```python
from build123d import *

# Parameters (mm, degrees)
EXTRUDE_1_DEPTH          = 5
EXTRUDE_2_DEPTH          = 15
EXTRUDE_2_DEPTH_BACK     = 5
SKETCH_3_R               = 3
CUT_EXTRUDE_1_DEPTH      = 3
SKETCH_4_R               = 2.1
CUT_EXTRUDE_2_DEPTH      = 10
CUT_EXTRUDE_3_DEPTH      = 86.718512573
CUT_EXTRUDE_3_DEPTH_BACK = 86.718512573
SKETCH_5_W               = 30
SKETCH_5_H               = 10
SKETCH_5_W_2             = 27.91179781
FILLET_1_R               = 3
CUT_EXTRUDE_4_DEPTH      = 88.407093534
CUT_EXTRUDE_4_DEPTH_BACK = 88.407093534
FILLET_2_R               = 3


with BuildPart() as part:
    # 草图1 → 凸台-拉伸1 (new body)
    with BuildSketch(Plane(origin=(0, 0, 0), x_dir=(1, 0, 0), z_dir=(0, 1, 0))):
        Polygon((0, 44.204391892), (-30, 44.204391892), (-30, -33.795608108), (0, -33.795608108), (30, -33.795608108), (30, 44.204391892), align=None)
    extrude(amount=EXTRUDE_1_DEPTH)

    # 草图2 → 凸台-拉伸2 (add, two sides: drawn at the far end of the back side and taken through both)
    with BuildSketch(Plane(origin=(0, 5, 0), x_dir=(1, 0, 0), z_dir=(0, 1, 0)).offset(-EXTRUDE_2_DEPTH_BACK)):
        Polygon((-30, -33.795608108), (-34, -33.795608108), (-34, 48.204391892), (34, 48.204391892), (34, -33.795608108), (30, -33.795608108), (30, 44.204391892), (-30, 44.204391892), align=None)
    extrude(amount=EXTRUDE_2_DEPTH + EXTRUDE_2_DEPTH_BACK)

    # 草图3 → 切除-拉伸1 (cut)
    with BuildSketch(Plane(origin=(0, 5, 0), x_dir=(1, 0, 0), z_dir=(0, 1, 0))):
        with Locations(Location((-20, 31.204391892, 0), (0, 0, 270))):
            Circle(SKETCH_3_R)
        with Locations(Location((20, 31.204391892, 0), (0, 0, 270))):
            Circle(SKETCH_3_R)
        with Locations(Location((-20, -18.795608108, 0), (0, 0, 270))):
            Circle(SKETCH_3_R)
        with Locations(Location((20, -18.795608108, 0), (0, 0, 270))):
            Circle(SKETCH_3_R)
    extrude(amount=-CUT_EXTRUDE_1_DEPTH, mode=Mode.SUBTRACT)

    # 草图4 → 切除-拉伸2 (cut)
    with BuildSketch(Plane(origin=(0, 2, 0), x_dir=(1, 0, 0), z_dir=(0, 1, 0))):
        with Locations(Location((-20, 31.204391892, 0), (0, 0, 270))):
            Circle(SKETCH_4_R)
        with Locations(Location((20, 31.204391892, 0), (0, 0, 270))):
            Circle(SKETCH_4_R)
        with Locations(Location((20, -18.795608108, 0), (0, 0, 270))):
            Circle(SKETCH_4_R)
        with Locations(Location((-20, -18.795608108, 0), (0, 0, 270))):
            Circle(SKETCH_4_R)
    extrude(amount=-CUT_EXTRUDE_2_DEPTH, mode=Mode.SUBTRACT)

    # 草图5 → 切除-拉伸3 (cut, two sides: drawn at the far end of the back side and taken through both)
    with BuildSketch(Plane.ZY.offset(34).offset(-CUT_EXTRUDE_3_DEPTH_BACK)):
        with Locations((-26.680193, 12)):
            Rectangle(SKETCH_5_W, SKETCH_5_H)
        with Locations((15.275705905, 12)):
            Rectangle(SKETCH_5_W_2, SKETCH_5_H)
    extrude(amount=CUT_EXTRUDE_3_DEPTH + CUT_EXTRUDE_3_DEPTH_BACK, mode=Mode.SUBTRACT)

    # 圆角1
    fillet_1_edges = [part.edges().sort_by_distance(p)[0] for p in [
        (-32, 17, -41.680193),
        (32, 17, -41.680193),
        (-32, 17, -11.680193),
        (32, 17, -11.680193),
        (-32, 7, -11.680193),
        (32, 7, -11.680193),
        (-32, 7, -41.680193),
        (32, 7, -41.680193),
        (-32, 17, 1.319807),
        (32, 17, 1.319807),
        (-32, 17, 29.23160481),
        (32, 17, 29.23160481),
        (-32, 7, 29.23160481),
        (32, 7, 29.23160481),
        (-32, 7, 1.319807),
        (32, 7, 1.319807),
    ]]
    fillet(fillet_1_edges, radius=FILLET_1_R)

    # 草图6 → 切除-拉伸4 (cut, two sides: drawn at the far end of the back side and taken through both)
    with BuildSketch(Plane.XY.offset(-44.204391892).offset(-CUT_EXTRUDE_4_DEPTH_BACK)):
        Polygon((0, 18), (-26, 18), (-26, 8), (26, 8), (26, 18), align=None)
    extrude(amount=CUT_EXTRUDE_4_DEPTH + CUT_EXTRUDE_4_DEPTH_BACK, mode=Mode.SUBTRACT)

    # 圆角2
    fillet_2_edges = [part.edges().sort_by_distance(p)[0] for p in [
        (26, 18, -46.204391892),
        (26, 8, -46.204391892),
        (-26, 8, -46.204391892),
        (-26, 18, -46.204391892),
    ]]
    fillet(fillet_2_edges, radius=FILLET_2_R)


solid = part.part
```
Design review of the part built by this model. Coordinates are the model's own, in mm. A direction names the side the tool comes from. Round coordinates to 2 decimals unless told otherwise and drop trailing zeros. Order: outer loops, then holes, each group sorted by start corner. A loop starts at its lowest first (then second) coordinate and runs counter-clockwise, first axis right, second up. Notation, with made-up numbers: (37.25, 59.25) - (59.25, 59.25) arc R11 cw to (59.25, 69.25) - close; hole circle Ø6 at (32, 76). An arc over 180 degrees is marked (long way). Return JSON: item names as keys, results as strings.
Q1. Consider section D-D on x = -20. Write out the cut boundary in (y, z), plus the area to 3 significant figures.
Computed values:
{"outline": "(0, -48.2) - (8, -48.2) - (8, -44.2) - (5, -44.2) - (5, -34.2) - (2, -34.2) - (2, -33.3) - (0, -33.3) - close; (0, -29.1) - (2, -29.1) - (2, -28.2) - (5, -28.2) - (5, 15.8) - (2, 15.8) - (2, 16.7) - (0, 16.7) - close; (0, 20.9) - (2, 20.9) - (2, 21.8) - (5, 21.8) - (5, 33.8) - (0, 33.8) - close; (18, -48.2) - (20, -48.2) - (20, -44.2) - (18, -44.2) - close", "area": "377 mm2"}
Q2. Consider section A-A on x = 15.5. Write out the cut boundary in (y, z).
Computed values:
{"outline": "(0, -48.2) - (8, -48.2) - (8, -44.2) - (5, -44.2) - (5, 33.8) - (0, 33.8) - close; (18, -48.2) - (20, -48.2) - (20, -44.2) - (18, -44.2) - close"}
Q3. The part is to be moulded in two halves that separate along X. For faces 5 (the cylindrical face through (25.1, 8.86, -46.18)), 6 (the cylindrical face through (21.42, 1.01, 17.25)), 7 (the cylindrical face through (31.972, 16.145, 28.329)), say which applies: pulls with the +X half, pulls with the -X half, needs draft (parallel to the pull), parting line crosses it, or undercut.
Computed values:
{"face 5": "undercut", "face 6": "undercut", "face 7": "needs draft"}
Q4. Consider section C-C on y = 12.25. Write out the cut boundary in (x, z).
Computed values:
{"outline": "(-34, -48.2) - (-26, -48.2) - (-26, -44.2) - (-30, -44.2) - (-30, -41.68) - (-34, -41.68) - close; (-34, -11.68) - (-30, -11.68) - (-30, 1.32) - (-34, 1.32) - close; (-34, 29.23) - (-30, 29.23) - (-30, 33.8) - (-34, 33.8) - close; (26, -48.2) - (34, -48.2) - (34, -41.68) - (30, -41.68) - (30, -44.2) - (26, -44.2) - close; (30, -11.68) - (34, -11.68) - (34, 1.32) - (30, 1.32) - close; (30, 29.23) - (34, 29.23) - (34, 33.8) - (30, 33.8) - close"}
Q5. For pin 1 Ø2 at (x, z) = (7, -19.5) entering from +Y; pin 2 Ø4 at (x, z) = (-20, -31.2) entering from +Y; pin 3 Ø5 at (x, z) = (20, 18.8) entering from +Y, all flat-tipped, find the tip position at first contact; note any pin that passes through.
Computed values:
{"pin 1": "stops at y = 5", "pin 2": "passes through", "pin 3": "stops at y = 2"}
Q6. Machinability: for faces 1 (the flat face through (-21, 2, -29)), 2 (the flat face through (0, 5, -6)), 3 (the cylindrical face through (25.14, 17.1, -46.18)), 4 (the cylindrical face through (-32.03, 7.9, -12.54)), which of the approach directions +Z, -Z, +X, -X, +Y, -Y give a long, thin tool a straight path to every point of the face, cutting with its end or side? Answer none if there is none.
Computed values:
{"face 1": "+Y", "face 2": "+Z, +Y", "face 3": "+Z, -Z", "face 4": "+X, -X"}
Q7. Wall thickness on L1, parallel to X at y = 17, z = -1; L2, parallel to Y at x = -24, z = -31; L3, parallel to Z at x = -21.5, y = 7: over which ranges is each line inside the solid? List them lowest first. Write a range as [from, to].
Computed values:
{"L1": "x = [-34, -30], [30, 34]", "L2": "y = [0, 5]", "L3": "z = [-48.2, -44.2]"}
Q8. Consider section B-B on z = -37.5. Write out the cut boundary in (x, y), plus the area to 3 significant figures.
Computed values:
{"outline": "(-34, 0) - (34, 0) - (34, 7) - (30, 7) - (30, 5) - (-30, 5) - (-30, 7) - (-34, 7) - close; (-34, 17) - (-30, 17) - (-30, 20) - (-34, 20) - close; (30, 17) - (34, 17) - (34, 20) - (30, 20) - close", "area": "380 mm2"}
